from build123d import *

# Parameters (mm, degrees)
F0_R      = 17.5
F1_DEPTH  = 60
F2_R      = 22.5
F3_DEPTH  = 40
F5_DEPTH  = 40
F7_D      = 3
F8_R      = 1.5
F9_DEPTH  = 5
F10_R     = 10
F11_DEPTH = 13
F12_R     = 4
F13_DEPTH = 22
F15_D     = 3
F15_DEPTH = 10
F15_TIP   = 0.9012909285
F16_R     = 2
F17_DEPTH = 12.5


with BuildPart() as f1:
    # F0 (on Front) → F1 (new body)
    with BuildSketch(Plane.XZ):
        Circle(F0_R)
    extrude(amount=F1_DEPTH)

    # F2 (on face) → F3 (join)
    with BuildSketch(Plane.XZ.offset(60)):
        Circle(F2_R)
    extrude(amount=F3_DEPTH)

    # F4 (on face) → F5 (join)
    with BuildSketch(Plane.XZ.offset(100)):
        with BuildLine():
            Line((4, -22.1415898255), (-4, -22.1415898255))
            ThreePointArc((-4, -22.1415898255), (0, -26.1415898255), (4, -22.1415898255))
        make_face()
        with BuildLine():
            Line((17.175179269, 14.5348965279), (21.175179269, 7.6066932976))
            ThreePointArc((21.175179269, 7.6066932976), (22.6392808842, 13.0707949127), (17.175179269, 14.5348965279))
        make_face()
        with BuildLine():
            Line((-21.175179269, 7.6066932976), (-17.175179269, 14.5348965279))
            ThreePointArc((-17.175179269, 14.5348965279), (-22.6392808842, 13.0707949127), (-21.175179269, 7.6066932976))
        make_face()
    extrude(amount=-F5_DEPTH)

    # F7 (through all)
    with Locations(Plane.XZ.offset(100)):
        with Locations((-19.0525588833, 11), (0, -22), (19.0525588833, 11)):
            Hole(F7_D / 2)

    # F8 (on face) → F9 (join)
    with BuildSketch(Plane.XZ.offset(100)):
        with BuildLine():
            Line((-3, 26.299103121), (-3, 22.299103121))
            Line((-3, 22.299103121), (3, 22.299103121))
            Line((3, 22.299103121), (3, 26.299103121))
            ThreePointArc((3, 26.299103121), (0, 29.299103121), (-3, 26.299103121))
        make_face()
        with Locations((0, 26.299103121)):
            Circle(F8_R, mode=Mode.SUBTRACT)
        with BuildLine():
            Line((-20.8115897844, -8.5514753491), (-24.2756913995, -10.5514753491))
            ThreePointArc((-24.2756913995, -10.5514753491), (-25.3737676109, -14.6495515605), (-21.2756913995, -15.7476277718))
            Line((-21.2756913995, -15.7476277718), (-17.8115897844, -13.7476277718))
            Line((-17.8115897844, -13.7476277718), (-20.8115897844, -8.5514753491))
        make_face()
        with Locations((-22.7756913995, -13.1495515605)):
            Circle(F8_R, mode=Mode.SUBTRACT)
        with BuildLine():
            Line((17.8115897844, -13.7476277718), (21.2756913995, -15.7476277718))
            ThreePointArc((21.2756913995, -15.7476277718), (25.3737676109, -14.6495515605), (24.2756913995, -10.5514753491))
            Line((24.2756913995, -10.5514753491), (20.8115897844, -8.5514753491))
            Line((20.8115897844, -8.5514753491), (17.8115897844, -13.7476277718))
        make_face()
        with Locations((22.7756913995, -13.1495515605)):
            Circle(F8_R, mode=Mode.SUBTRACT)
    extrude(amount=-F9_DEPTH)

    # F10 (on face) → F11 (join)
    with BuildSketch(Plane.XZ.offset(100)):
        Circle(F10_R)
    extrude(amount=F11_DEPTH)

    # F12 (on face) → F13 (join)
    with BuildSketch(Plane.XZ.offset(113)):
        Circle(F12_R)
    extrude(amount=F13_DEPTH)

    # F15
    with Locations(Plane.XZ.offset(135)):
        with Locations((0, 0)):
            Hole(F15_D / 2, depth=F15_DEPTH)
            with Locations((0, 0, -(F15_DEPTH + F15_TIP / 2))):  # 118° drill point
                Cone(0, F15_D / 2, F15_TIP, mode=Mode.SUBTRACT)

    # F16 (on Top) → F17 (cut, symmetric)
    with BuildSketch(Plane.XY):
        with Locations((0, -118)):
            Circle(F16_R)
    extrude(amount=F17_DEPTH, both=True, mode=Mode.SUBTRACT)


solid = f1.part
Verification items for the finished model (mm, model axes). A direction names the side the tool comes from. Give positions to 0.01 mm unless a question says otherwise; leave off trailing zeros. Order: outer loops, then holes, each group sorted by start corner. A loop starts at its lowest first (then second) coordinate and runs counter-clockwise, first axis right, second up. Notation, with made-up numbers: M 65.25,5 L 81.25,5 A11 ccw 81.25,10 Z; hole C 40,-6.75 d11. An arc over 180 degrees is marked long. Use one line per item in the form item = value. Start each with the question number.
Q1. Mould release check, pull along Z, two halves, no side actions. Record for faces 1 (the flat face through (-16, -60, -9)), 2 (the cylindrical face through (3.695, -123.846, -1.532)), 3 (the cylindrical face through (-22.59, -80.28, 13.15)): +Z half, -Z half, draft (parallel to the pull), parting line (faces both ways), or undercut.
Q2. Go/stop test with flat-tipped pins: pin 1 Ø10 at (x, y) = (15.5, -67) entering from -Z; pin 2 Ø1.8 at (x, z) = (0, -22) entering from -Y; pin 3 Ø8.5 at (x, z) = (22.5, -12) entering from +Y; pin 4 Ø8 at (y, z) = (-53, -13) entering from -X. Record where each tip stops, or that it passes through.
Q3. Section check A-A (y = -109.5). Enter the section's corners in (x, z).
Q4. Access from +Z, -Z, +X, -X, +Y, -Y to the whole of each face (thin tool, end or side, straight path). Record for faces 4 (the flat face through (-3, -98, 24)), 5 (the flat face through (-19.568, -97.535, -14.762)), 6 (the cylindrical face through (1.5, -129.93, 0.07)), 7 (the flat face through (21, -95, -13)).
Q5. Section check B-B (y = -40.5). Enter the section's corners in (x, z).
Q6. Scan lines: line 1 along Z through (x, y) = (0, -84); line 2 along X through (y, z) = (-46, -1); line 3 along Y through (x, z) = (22, 0). Record each from-to range of solid material in increasing order. Write a range as [from, to].
Evaluation:
q1.face_1 = draft
q1.face_2 = parting line
q1.face_3 = undercut
q2.pin_1 = -19.9
q2.pin_2 = through
q2.pin_3 = -60
q2.pin_4 = -15.01
q3.outline = C 0,0 d20
q4.face_4 = +Z, -X, +Y, -Y
q4.face_5 = -Z, +Y, -Y
q4.face_6 = -Y
q4.face_7 = -Z, +X, +Y
q5.outline = C 0,0 d35
q6.line_1 = [-26.14, -23.5], [-20.5, 22.5]
q6.line_2 = [-17.47, 17.47]
q6.line_3 = [-100, -60]
